```python
from build123d import *

# Parameters (mm, degrees)
BOSS_EXTRUDE1_DEPTH     = 12.7
F_1_4_CLEARANCE_HOLE1_D = 6.7564
M8_CLEARANCE_HOLE1_D    = 8.4
CHAMFER1_SIZE           = 1


with BuildPart() as part:
    # Sketch1 → Boss-Extrude1 (new, symmetric)
    with BuildSketch(Plane(origin=(0, 0, 0), x_dir=(0, 0, -1), z_dir=(1, 0, 0))):
        Polygon((-44.45, 241.3), (-12.7, 241.3), (-12.7, 260.35), (-25.4, 260.35), (-25.4, 298.45), (-12.7, 298.45), (-12.7, 317.5), (-44.45, 317.5), align=None)
    extrude(amount=BOSS_EXTRUDE1_DEPTH, both=True)

    # 1/4 Clearance Hole1 (through all)
    with Locations(Plane(origin=(12.7, 0, 0), x_dir=(0, 0, -1), z_dir=(1, 0, 0))):
        with Locations((-33.4, 304.4), (-33.4, 254.4)):
            Hole(F_1_4_CLEARANCE_HOLE1_D / 2)

    # M8 Clearance Hole1 (through all)
    with Locations(Plane(origin=(0, 0, 25.4), x_dir=(-1, 0, 0), z_dir=(0, 0, -1))):
        with Locations((0, 279.4)):
            Hole(M8_CLEARANCE_HOLE1_D / 2)

    # Chamfer1
    chamfer1_edges = [part.edges().sort_by_distance(p)[0] for p in [
        (12.7, 254.4, 30.0218),
        (-12.7, 254.4, 30.0218),
        (12.7, 304.4, 30.0218),
        (-12.7, 304.4, 30.0218),
        (-4.2, 279.4, 25.4),
        (-4.2, 279.4, 44.45),
    ]]
    chamfer(chamfer1_edges, length=CHAMFER1_SIZE)


solid = part.part
```
Model file for the job. Use its own axes, mm. A direction names the side the tool comes from. Coordinates: 2 decimals unless noted, no trailing zeros. Loops run counter-clockwise (first coordinate to the right, second up) from the corner with the lowest first, then second, coordinate; pieces in that order, holes last. Notation, with made-up numbers: (-17.75, 8) - (31.25, 8) arc R32 cw to (31.25, 37) - close; hole circle Ø1 at (22, 10). An arc over 180 degrees is marked (long way). Answer as a JSON object with one key per item and string values. Group by question number.
(1) Cut at A-A (y = 304.4). Give the cut face in (x, z), then the cut area to 3 significant figures.
(2) Two-plate mould, pull along X, no slides. Class faces 1 (the face through (0, 298.45, 19)), 2 (the face through (-0.91, 275.3, 35.04)), 3 (the face through (-12.7, 280, 32)): released by +X, released by -X, zero draft, split by the parting line, or undercut.
(3) Cut at B-B (x = 0). Give the cut face in (y, z), then the cut area to 3 significant figures.
(4) Probe line 1 along Y through (x, z) = (4.5, 33.4); line 2 along Y through (x, z) = (0, 38.5); line 3 along Z through (x, y) = (4, 254.4). List the from-to ranges inside material, lowest first.
(5) Tool access for faces 4 (the face through (-0.16, 307.75, 32.96)), 5 (the face through (0, 260.35, 19)): list every direction of +Z, -Z, +X, -X, +Y, -Y with a clear straight run to the whole face (end or side of a thin tool).
(6) Cut at D-D (x = -8.75). Give the cut face in (y, z), then the cut area to 3 significant figures.
(7) Cut at C-C (z = 24.5). Give the cut face in (x, y), then the cut area to 3 significant figures.
(8) Flat gauge pins, fed straight in: pin 1 (7.5 mm diameter, centred on x = -0.5, y = 279.5, fed in from -Z); pin 2 (9.5 mm diameter, centred on x = 0, y = 279.4, fed in from +Z). Where does each tip first touch, or does it go through?
Geometry says:
{
 "1": {"outline": "(-12.7, 12.7) - (12.7, 12.7) - (12.7, 29.02) - (11.7, 30.02) - (-11.7, 30.02) - (-12.7, 29.02) - close; (-12.7, 37.78) - (-11.7, 36.78) - (11.7, 36.78) - (12.7, 37.78) - (12.7, 44.45) - (-12.7, 44.45) - close", "area": "633 mm^2"},
 "2": {"face 1": "zero draft", "face 2": "undercut", "face 3": "released by -X"},
 "3": {"outline": "(241.3, 12.7) - (260.35, 12.7) - (260.35, 25.4) - (274.2, 25.4) - (275.2, 26.4) - (275.2, 43.45) - (274.2, 44.45) - (241.3, 44.45) - close; (283.6, 26.4) - (284.6, 25.4) - (298.45, 25.4) - (298.45, 12.7) - (317.5, 12.7) - (317.5, 44.45) - (284.6, 44.45) - (283.6, 43.45) - close; hole circle Ø6.76 at (254.4, 33.4); hole circle Ø6.76 at (304.4, 33.4)", "area": "1,700 mm^2"},
 "4": {"line 1": "y = 241.3 to 251.02, 257.78 to 301.02, 307.78 to 317.5", "line 2": "y = 241.3 to 275.2, 283.6 to 317.5", "line 3": "z = 12.7 to 30.02, 36.78 to 44.45"},
 "5": {"face 4": "+X, -X", "face 5": "-Z, +X, -X"},
 "6": {"outline": "(241.3, 12.7) - (260.35, 12.7) - (260.35, 25.4) - (298.45, 25.4) - (298.45, 12.7) - (317.5, 12.7) - (317.5, 44.45) - (241.3, 44.45) - close; hole circle Ø6.76 at (254.4, 33.4); hole circle Ø6.76 at (304.4, 33.4)", "area": "1,860 mm^2"},
 "7": {"outline": "(-12.7, 241.3) - (12.7, 241.3) - (12.7, 260.35) - (-12.7, 260.35) - close; (-12.7, 298.45) - (12.7, 298.45) - (12.7, 317.5) - (-12.7, 317.5) - close", "area": "968 mm^2"},
 "8": {"pin 1": "stops at z = 26.34", "pin 2": "stops at z = 44"}
}
